```python
from build123d import *

# Parameters (mm, degrees)
SKETCH1_W           = 20
SKETCH1_H           = 140
BOSS_EXTRUDE1_DEPTH = 10
CHAMFER1_SIZE       = 2
SKETCH2_R           = 3
CUT_EXTRUDE1_DEPTH  = 11


with BuildPart() as part:
    # Sketch1 → Boss-Extrude1 (new body)
    with BuildSketch(Plane.XY):
        Rectangle(SKETCH1_W, SKETCH1_H)
    extrude(amount=BOSS_EXTRUDE1_DEPTH)

    # Chamfer1
    chamfer1_edges = [part.edges().sort_by_distance(p)[0] for p in [
        (10, 0, 0),
        (10, 0, 10),
    ]]
    chamfer(chamfer1_edges, length=CHAMFER1_SIZE)

    # Sketch2 → Cut-Extrude1 (cut, through all)
    with BuildSketch(Plane.XY.offset(10)):
        with Locations((-4, 55)):
            Circle(SKETCH2_R)
        with Locations((-4, 0)):
            Circle(SKETCH2_R)
        with Locations((-4, -55)):
            Circle(SKETCH2_R)
    extrude(amount=-CUT_EXTRUDE1_DEPTH, mode=Mode.SUBTRACT)


solid = part.part
```
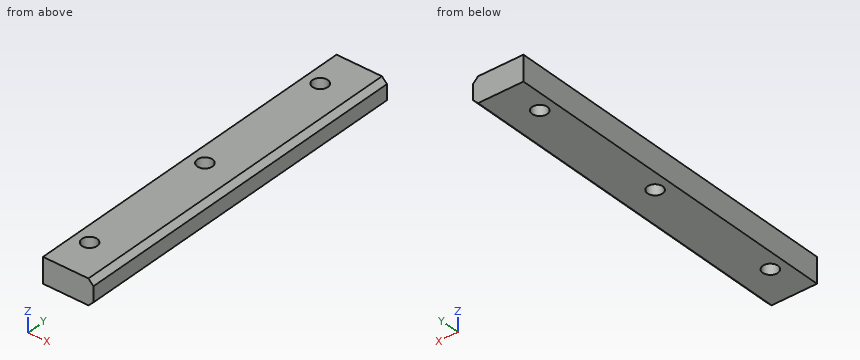
CAD build for the part. Positions are in the model's coordinates, mm. Round coordinates to 2 decimals unless told otherwise and drop trailing zeros. Order: outer loops, then holes, each group sorted by start corner. A loop starts at its lowest first (then second) coordinate and runs counter-clockwise, first axis right, second up.
Q1. Wall check: L1, parallel to Y at x = -4, z = 2.25; L2, parallel to Y at x = -5.5, z = 5.5; L3, parallel to X at y = -53, z = 3.25. Give the ranges that are in metal, low to high.
Q2. Drop a flat-ended pin along its axis: pin 1 (5.5 mm diameter, centred on x = -4, y = -55, fed in from +Z). Give the stop position or say it passes through.
Q3. Slice it at B-B (x = -4). Write the cut outline in (y, z), and give its area (3 significant figures).
Q4. Slice it at A-A (y = 55). Write the cut outline in (x, z), and give its area (3 significant figures).
Q5. Slice it at C-C (y = 25.5). Write the cut outline in (x, z).
Results below:
1. L1: y = -70 to -58, -52 to -3, 3 to 52, 58 to 70
1. L2: y = -70 to -57.6, -52.4 to -2.6, 2.6 to 52.4, 57.6 to 70
1. L3: x = -10 to -6.24, -1.76 to 10
2. pin 1: passes through
3. outline: (-70, 0) - (-58, 0) - (-58, 10) - (-70, 10) - close; (-52, 0) - (-3, 0) - (-3, 10) - (-52, 10) - close; (3, 0) - (52, 0) - (52, 10) - (3, 10) - close; (58, 0) - (70, 0) - (70, 10) - (58, 10) - close
3. area: 1,220 mm2
4. outline: (-10, 0) - (-7, 0) - (-7, 10) - (-10, 10) - close; (-1, 0) - (8, 0) - (10, 2) - (10, 8) - (8, 10) - (-1, 10) - close
4. area: 136 mm2
5. outline: (-10, 0) - (8, 0) - (10, 2) - (10, 8) - (8, 10) - (-10, 10) - close
